from build123d import *

# Parameters (mm, degrees)
ESBO_O2_R                     = 11
RESSALTO_EXTRUS_O1_DEPTH      = 180
ESBO_O11_R                    = 6
RESSALTO_EXTRUS_O4_DEPTH      = 41
CORTE_EXTRUS_O1_START         = -1
ESBO_O15_R                    = 6
CORTE_EXTRUS_O1_DEPTH         = 1
FURO_ROSCADO_DE_M8X1_01_D     = 7
FURO_ROSCADO_DE_M8X1_01_DEPTH = 35
FURO_ROSCADO_DE_M8X1_01_TIP   = 2.103012167


with BuildPart() as part:
    # Esboço2 → Ressalto-extrusão1 (new body)
    with BuildSketch(Plane.XY):
        with Locations(Location((0, 0, 0), (0, 0, 180))):
            Circle(ESBO_O2_R)
    extrude(amount=RESSALTO_EXTRUS_O1_DEPTH)

    # Esboço11 → Ressalto-extrusão4 (add)
    with BuildSketch(Plane.XY.offset(180)):
        Circle(ESBO_O11_R)
    extrude(amount=RESSALTO_EXTRUS_O4_DEPTH)

    # Esboço15 → Corte-extrusão1 (cut)
    with BuildSketch(Plane.XY.offset(221).offset(CORTE_EXTRUS_O1_START)):
        Circle(ESBO_O15_R)
    extrude(amount=CORTE_EXTRUS_O1_DEPTH, mode=Mode.SUBTRACT)

    # Furo roscado de M8x1.01
    with Locations(Plane(origin=(0, 0, 0), x_dir=(-1, 0, 0), z_dir=(0, 0, -1))):
        with Locations((0, 0)):
            Hole(FURO_ROSCADO_DE_M8X1_01_D / 2, depth=FURO_ROSCADO_DE_M8X1_01_DEPTH)
            with Locations((0, 0, -(FURO_ROSCADO_DE_M8X1_01_DEPTH + FURO_ROSCADO_DE_M8X1_01_TIP / 2))):  # 118° drill point
                Cone(0, FURO_ROSCADO_DE_M8X1_01_D / 2, FURO_ROSCADO_DE_M8X1_01_TIP, mode=Mode.SUBTRACT)


solid = part.part
Verification items for the finished model (mm, model axes). A direction names the side the tool comes from. Round coordinates to 2 decimals unless told otherwise and drop trailing zeros. Order: outer loops, then holes, each group sorted by start corner. A loop starts at its lowest first (then second) coordinate and runs counter-clockwise, first axis right, second up.
1. Go/stop test with flat-tipped pins: P1, Ø1.5, axis at y = 4, z = 146.5, coming from the -X side; P2, Ø10, axis at y = -7, z = 190.5, coming from the -X side; P3, Ø8, axis at y = 4.5, z = 85, coming from the +X side. Record where each tip stops, or that it passes through.
Final values:
P1: stops at x = -10.51
P2: stops at x = -5.66
P3: stops at x = 10.99
2. Access from +Z, -Z, +X, -X, +Y, -Y to the whole of each face (thin tool, end or side, straight path). Record for faces 4 (the flat face through (0, 0, 220)), 5 (the flat face through (-5, 5, 180)).
Final values:
face 4: +Z, +X, -X, +Y, -Y
face 5: +Z
3. Section check A-A on z = 47.5. Record the cut outline in (x, y), then the cut area to 3 significant figures.
Final values:
outline: circle Ø22 at (0, 0)
area: 380 mm2
4. Thickness scan on L1, parallel to Y at x = 0, z = 10.5; L2, parallel to Z at x = 2.25, y = 7.5; L3, parallel to Y at x = -0.5, z = 172. Record the ranges inside material, lowest first.
Final values:
L1: y = -11 to -3.5, 3.5 to 11
L2: z = 0 to 180
L3: y = -10.99 to 10.99
5. Section check B-B on z = 197.5. Record the cut outline in (x, y).
Final values:
outline: circle Ø12 at (0, 0)
6. Release check for a two-part mould opening along X. For faces 1 (the cylindrical face through (-6, 0, 200)), 2 (the flat face through (3, -3, 0)), 3 (the cylindrical face through (3.233, -1.341, 17.745)) record: +X half, -X half, draft (parallel to the pull), parting line (faces both ways), or undercut.
Final values:
face 1: parting line
face 2: draft
face 3: undercut
